Autodesk Inventor part; units mm, degrees
ref_plane "YZ Plane" through (0, 0, 0) normal (1, 0, 0) x (0, 1, 0)
ref_plane "XZ Plane" through (0, 0, 0) normal (0, 1, 0) x (-1, 0, 0)
ref_plane "XY Plane" through (0, 0, 0) normal (0, 0, 1) x (1, 0, 0)
sketch "Sketch1" plane through (0, 0, 0) normal (1, 0, 0) x (0, 1, 0)
  line L0 (0, 0) -> (0, -68)
  line L1 (0, -68) -> (0, -60)
  line L2 (0, 0) -> (0, -8)
  circle A0 centre (0, -4) radius 4
  circle A1 centre (0, -64) radius 4
  circle A2 centre (0, -64) radius 7.5
  circle A3 centre (0, -4) radius 7.5
  circle A4 centre (0, -4) radius 10
  circle A5 centre (0, -64) radius 10
  line L3 (10, -4) -> (10, -64)
  dimension "d5" = 20
  dimension "d6" = 20
  dimension "d0" = 68
  dimension "d1" = 8
  dimension "d2" = 8
  dimension "d3" = 15
  dimension "d4" = 15
extrude "Extrusion1" add sketch "Sketch1" along normal blind 15.24 contours A4 | A5
sketch "Sketch2" plane through (0, 0, -4) normal (-1, 0, 0) x (0, 0, 1)
  circle A0 centre (0, 0) radius 10
  line L0 (0, 10) -> (-60, 10)
  circle A1 centre (-60, 0) radius 10
  line L1 (-50, 0) -> (-10, 0)
  point P0 (4, 0)
extrude "Extrusion2" add sketch "Sketch2" along normal blind 2.54
sketch "Sketch3" plane through (0, 0, -4) normal (1, 0, 0) x (0, 0, -1)
  line L0 (0, 10) -> (60, 10)
  arc A0 (10, 0) -> (0, 10) centre (0, 0) ccw
  line L1 (50, 0) -> (10, 0)
  arc A1 (60, 10) -> (50, 0) centre (60, 0) ccw
  line L2 (0, 10) -> (60, 10)
  point P0 (-4, 0)
extrude "Extrusion3" add sketch "Sketch3" along normal up to surface (15.24 mm away)
sketch "Sketch4" plane through (-2.54, 0, -14) normal (0, -1, 0) x (1, 0, 0)
  line L0 (0, 0) -> (17.78, 0)
  line L1 (17.78, 0) -> (17.78, -15.875)
  line L2 (17.78, -40) -> (0, -40)
  line L3 (17.78, -40) -> (17.78, 0)
  arc A0 (17.78, -24.125) -> (17.78, -40.1897) centre (17.78, -32.1574) ccw
  line L4 (17.78, 0) -> (17.78, -15.875)
  arc A1 (17.78, 0) -> (17.78, -15.875) centre (17.78, -7.9375) ccw
  line L5 (17.78, -24.125) -> (17.78, -40.1897)
  point P0 (2.54, 14)
  dimension "d13" = 15.875
  dimension "d16" = 15.875
extrude "Extrusion4" cut sketch "Sketch4" against normal blind 2.54
sketch "Sketch5" plane through (-2.54, 2.54, -14) normal (0, -1, 0) x (1, 0, 0)
  line L0 (17.78, 0) -> (17.78, 20)
  line L1 (17.78, -24.125) -> (17.78, -15.875)
  arc A0 (17.78, 0) -> (17.78, -15.875) centre (17.78, -7.9375) ccw
  line L2 (0, 0) -> (17.78, 0)
  line L3 (0, -40) -> (0, 0)
  line L4 (16.0445, -40) -> (0, -40)
  arc A1 (17.78, -24.125) -> (16.0445, -40) centre (17.78, -32.1574) ccw
  line L5 (17.78, -24.125) -> (17.78, -15.875)
  line L6 (17.78, 0) -> (17.78, -15.875)
  line L7 (17.78, 10) -> (17.78, -50)
  line L8 (17.78, -60) -> (17.78, -40)
  line L9 (17.78, -24.125) -> (17.78, -40)
  circle A2 centre (17.78, -7.9375) radius 6
  circle A3 centre (17.78, -32.1574) radius 6
  point P0 (2.54, 14)
  dimension "d20" = 12
  dimension "d21" = 12
extrude "Extrusion5" cut sketch "Sketch5" against normal blind 6 contours A3 L7 | L7 A3 | A2 L6 | L6 A2
sketch "Sketch6" plane through (-2.54, 8.54, -14) normal (0, -1, 0) x (1, 0, 0)
  line L0 (17.78, -26.1574) -> (17.78, -38.1574)
  circle A0 centre (17.78, -32.1574) radius 8.0324
  line L1 (17.78, -1.9375) -> (17.78, -13.9375)
  arc A1 (17.78, -1.9375) -> (17.78, -13.9375) centre (17.78, -7.9375) ccw
  circle A2 centre (17.78, -7.9375) radius 7.9375
  point P0 (2.54, 14)
extrude "Extrusion6" cut sketch "Sketch6" against normal blind 6 contours A0 | L1 A1 | A2
sketch "Sketch7" plane through (15.24, 0, 0) normal (1, 0, 0) x (0, 0, -1)
  line L0 (29.875, 10) -> (38.125, 10)
  arc A0 (4, 10) -> (14, 0) centre (4, 0) ccw
  line L1 (34, 10) -> (14, 10)
  line L2 (14, 10) -> (14, 0)
  line L3 (14, 0) -> (34, 0)
  line L4 (34, 0) -> (34, 10)
  point P0 (0, 0)
extrude "Extrusion7" add sketch "Sketch7" against normal blind 12
sketch "Sketch8" plane through (15.24, 0, 0) normal (1, 0, 0) x (0, 0, -1)
  line L0 (54, 0) -> (14, 0)
  line L1 (34, 0) -> (14, 0)
  line L2 (14, 0) -> (14, -12.065)
  line L3 (14, -12.065) -> (34, -12.065)
  line L4 (34, -12.065) -> (34, 0)
  point P0 (0, 0)
  dimension "d28" = 12.065
extrude "Extrusion8" add sketch "Sketch8" against normal up to surface (17.78 mm away)
sketch "Sketch9" plane through (15.24, -12.065, -34) normal (0, -1, 0) x (1, 0, 0)
  line L0 (-17.78, 20) -> (0, 20)
  line L1 (0, 20) -> (0, 4.125)
  line L2 (0, 20) -> (0, 0)
  arc A0 (0, 20) -> (0, 4.125) centre (0, 12.0625) ccw
  point P0 (-15.24, 34)
  dimension "d31" = 15.875
  dimension "d32" = 7.9375
extrude "Extrusion9" cut sketch "Sketch9" against normal blind 3.81
sketch "Sketch10" plane through (15.24, -8.255, -34) normal (0, -1, 0) x (1, 0, 0)
  line L0 (0, 20) -> (0, 4.125)
  arc A0 (0, 20) -> (0, 4.125) centre (0, 12.0625) ccw
  circle A1 centre (0, 12.0625) radius 6
  point P0 (-15.24, 34)
  dimension "d35" = 12
extrude "Extrusion10" cut sketch "Sketch10" against normal blind 5.5 contours A1 L0 | L0 A1
sketch "Sketch11" plane through (15.24, -2.755, -34) normal (0, -1, 0) x (1, 0, 0)
  line L0 (0, 18.0625) -> (0, 6.0625)
  circle A0 centre (0, 12.0625) radius 7.9375
  point P0 (-15.24, 34)
extrude "Extrusion11" cut sketch "Sketch11" against normal blind 9
sketch "Sketch12" plane through (15.24, 6.245, -34) normal (0, -1, 0) x (1, 0, 0)
  line L0 (0, 20) -> (0, 4.125)
  circle A0 centre (0, 12.0625) radius 12.5
  point P0 (-15.24, 34)
  dimension "d40" = 25
extrude "Extrusion12" cut sketch "Sketch12" against normal blind 9
sketch "Sketch13" plane through (15.24, 0, 0) normal (1, 0, 0) x (0, 0, -1)
  line L0 (9.4375, 6.245) -> (9.4375, 10)
  line L1 (4, 10) -> (9.4375, 10)
  arc A0 (4, 10) -> (14, 0) centre (4, 0) ccw
  line L2 (14, 0) -> (14, 6.245)
  line L3 (14, 6.245) -> (9.4375, 6.245)
  circle A1 centre (4, 0) radius 7.5
  line L4 (14, -8.255) -> (14, -12.065)
  line L5 (14, -12.065) -> (2.7589, -9.9227)
  arc A2 (4, 10) -> (14, 0) centre (4, 0) ccw
  line L6 (14, 0) -> (14, -12.065)
  line L7 (14, -12.065) -> (14, 0)
  line L8 (14, -12.065) -> (14, 0)
  line L9 (14, 0) -> (8.3795, -7.0711)
  line L10 (8.3795, -7.0711) -> (2.7589, -9.9227)
  point P0 (0, 0)
extrude "Extrusion13" add sketch "Sketch13" against normal up to surface (17.78 mm away) contours L6 L4 L5 A0
sketch "Sketch14" plane through (-2.54, 0, -4) normal (-1, 0, 0) x (0, 0, 1)
  line L0 (-30, -12.065) -> (-10, -12.065)
  arc A0 (1.2411, -9.9227) -> (0, 10) centre (0, 0) ccw
  arc A1 (1.2411, -9.9227) -> (0, 10) centre (0, 0) ccw
  line L1 (0, 10) -> (-60, 10)
  arc A2 (-60, 10) -> (-50, 0) centre (-60, 0) ccw
  line L2 (-50, 0) -> (-30, 0)
  line L3 (-30, 0) -> (-30, -12.065)
  line L4 (-30, -12.065) -> (-10, -12.065)
  line L5 (-10, -12.065) -> (1.2411, -9.9227)
  line L6 (-30, -12.065) -> (-58.9174, -9.9412)
  arc A3 (-60, 10) -> (-50, 0) centre (-60, 0) ccw
  point P0 (4, 0)
extrude "Extrusion14" add sketch "Sketch14" against normal blind 2.54 contours L6 A2 L2 L3
sketch "Sketch15" plane through (0, 0, -4) normal (1, 0, 0) x (0, 0, -1)
  circle A0 centre (0, 0) radius 4.5
  circle A1 centre (60, 0) radius 7.5
  circle A2 centre (60, 0) radius 4.5
  point P0 (-4, 0)
  dimension "d47" = 9
  dimension "d48" = 9
extrude "Extrusion15" cut sketch "Sketch15" against normal blind 2.54 contours A0 | A2
sketch "Sketch16" plane through (15.24, 0, 0) normal (1, 0, 0) x (0, 0, -1)
  circle A0 centre (34.2867, 3.4117) radius 1.5
  point P0 (0, 0)
  dimension "d51" = 3
extrude "Extrusion16" cut sketch "Sketch16" against normal blind 70.8025
sketch "Sketch17" plane through (15.24, 0, 0) normal (1, 0, 0) x (0, 0, -1)
  circle A0 centre (56.0987, 6.4645) radius 1.5
  circle A1 centre (11.0664, -7.5602) radius 1.5
  point P0 (0, 0)
  dimension "d54" = 3
  dimension "d55" = 3
extrude "Extrusion17" cut sketch "Sketch17" against normal blind 70.8025
properties part number "Hotend holder V4"
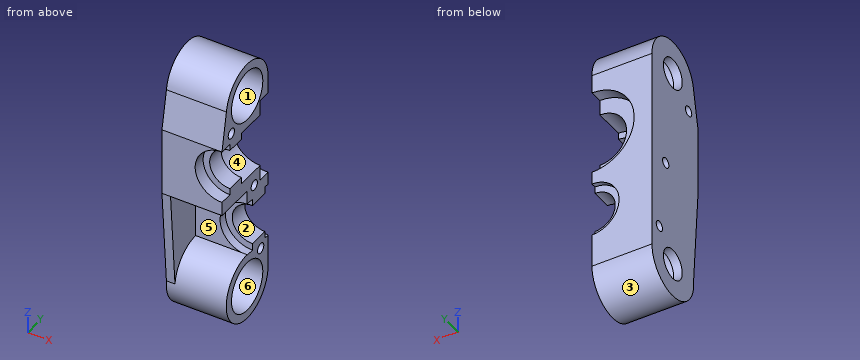
For this review, take the finished solid that the model builds, in its own axes (mm). Face numbers are marked on the shaded views. A direction names the side the tool comes from. Round coordinates to 2 decimals unless told otherwise and drop trailing zeros. Order: outer loops, then holes, each group sorted by start corner. A loop starts at its lowest first (then second) coordinate and runs counter-clockwise, first axis right, second up. Notation, with made-up numbers: (47, -38.75) -> (102, -38.75) arc R20 cw to (102, -4.75) -> close; hole circle Ø7 at (-22, 86.5). An arc over 180 degrees is marked (long way). Put each result on its own line as item: value.
Q1. Add section C-C on x = 12.75. State how many separate pieces and enclosed holes the cut face has, plus the area to 3 significant figures.
Check result:
separate pieces: 3
enclosed holes: 5
area: 499 mm2
Q2. Add section A-A on x = 5.5. Write out the cut boundary in (y, z) (1 decimal), plus the area to 3 significant figures.
Check result:
outline: (-12.1, -34) -> (0, -34) -> (0, -54) arc R10 ccw (long way) to (10, -64) -> (10, -29.8) -> (6.2, -29.8) -> (6.2, -14.1) -> (10, -14.1) -> (10, -4) arc R10 ccw to (-9.9, -2.8) -> (-12.1, -14) -> close; hole circle Ø3 at (-7.6, -11.1); hole circle Ø15 at (0, -64); hole circle Ø15 at (0, -4); hole circle Ø3 at (3.4, -34.3); hole circle Ø3 at (6.5, -56.1)
area: 912 mm2
Q3. For probe 1 along Z at (x, y) = (4.5, 3.5); probe 2 along Z at (x, y) = (14.5, 1.75); probe 3 along X at (y, z) = (-10.75, -48.5), list the stretches that pass through material, from the lowest coordinate up. Write a range as [from, to].
Check result:
probe 1: [-73.37, -70.63], [-57.37, -35.78], [-32.79, -10.63], [2.63, 5.37]
probe 2: [-73.85, -71.29], [-56.71, -54.16], [-38.16, -29.84], [-14.03, -11.29], [3.29, 5.85]
probe 3: [-2.54, 0]
Q4. Mouldability with a two-part tool opening along Y and no side actions: class the marked faces 1, 2 and 3 as pulls with the +Y half, pulls with the -Y half, needs draft (parallel to the pull), parting line crosses it, or undercut.
Check result:
face 1: undercut
face 2: needs draft
face 3: parting line crosses it
Q5. Add section B-B on z = -41.5. Write out the cut boundary in (x, y).
Check result:
outline: (-2.54, -11.51) -> (0, -11.51) -> (0, 0) -> (8.7, 0) -> (8.7, 2.54) -> (11.46, 2.54) -> (11.46, 8.54) -> (8.7, 8.54) -> (8.7, 10) -> (-2.54, 10) -> close
Q6. Add section D-D on z = -26. Write out the cut boundary in (x, y) (3 decimals).
Check result:
outline: (-2.54, -12.065) -> (8.421, -12.065) -> (8.421, -8.255) -> (10.825, -8.255) -> (10.825, -2.755) -> (8.421, -2.755) -> (8.421, 6.245) -> (3.419, 6.245) -> (3.419, 10) -> (-2.54, 10) -> close
Q7. Insertion check: pin 1 Ø2.5 at (y, z) = (-7.56, -11.07) entering from +X; pin 2 Ø5 at (y, z) = (-6.5, -51) entering from +X; pin 3 Ø1 at (y, z) = (3, -44.5) entering from +X; pin 4 Ø6.5 at (x, z) = (13, -18.5) entering from +Y (3 decimals). Each pin has a flat end and moves straight along its axis. Give the tip position at first contact, or say it passes through.
Check result:
pin 1: through
pin 2: x = 0
pin 3: x = 9.64
pin 4: y = -2.755
Q8. Machinability: for the marked faces 4, 5 and 6, which of the approach directions +Z, -Z, +X, -X, +Y, -Y give a long, thin tool a straight path to every point of the face, cutting with its end or side? Answer none if there is none.
Check result:
face 4: +X, +Y
face 5: +X, -Y
face 6: +X
